```python
from build123d import *

# Parameters (mm, degrees)
BOSS_EXTRUDE1_DEPTH = 1.5


with BuildPart() as part:
    # Sketch2 → Boss-Extrude1 (new body, symmetric)
    with BuildSketch(Plane.XY):
        with BuildLine():
            Line((-15.000000098, -155.000001017), (-1.550000098, -155.000001017))
            Line((-1.550000098, -155.000001017), (-1.550000098, 164.999998983))
            Line((-1.550000098, 164.999998983), (1.549999902, 164.999998983))
            Line((1.549999902, 164.999998983), (1.549999902, -155.000001017))
            Line((1.549999902, -155.000001017), (14.999999902, -155.000001017))
            Line((14.999999902, -155.000001017), (14.999999902, 154.999998983))
            ThreePointArc((14.999999902, 154.999998983), (1.936e-06, 170.000001017), (-15.000000098, 155.000003052))
            Line((-15.000000098, 155.000003052), (-15.000000098, -155.000001017))
        make_face()
    extrude(amount=BOSS_EXTRUDE1_DEPTH, both=True)


solid = part.part
```
Part model, mm, in its own coordinate system. Give positions to 0.01 mm unless a question says otherwise; leave off trailing zeros. Write each loop counter-clockwise with the first axis right and the second up, starting at its lowest first coordinate (ties: lowest second). Pieces come first, ordered by that corner, then holes. Notation, with made-up numbers: (-10, 49.25) -> (7, 49.25) arc R14 cw to (7, 54.25) -> close; hole circle Ø10 at (53, 12.5). An arc over 180 degrees is marked (long way). Put each result on its own line as item: value. Start each with the question number.
Item 1: Cut at A-A (y = -106). List the corners of the cut face in (x, z), then the cut area to 3 significant figures.
Item 2: Cut at B-B (z = -1). List the corners of the cut face in (x, y), then the cut area to 3 significant figures.
Item 3: Pin check, flat tips, straight feed: pin 1 Ø1 at (x, z) = (-11.5, 0) entering from +Y; pin 2 Ø0.9 at (x, z) = (0.5, 0.5) entering from -Y. Stop position of each tip, or through.
Item 4: Wall check: L1, parallel to X at y = -88, z = 0.15; L2, parallel to Y at x = 0.5, z = 0.8; L3, parallel to Y at x = 3, z = 0.1. Give the ranges that are in metal, low to high. Write a range as [from, to].
Answer list:
1. outline: (-15, -1.5) -> (-1.55, -1.5) -> (-1.55, 1.5) -> (-15, 1.5) -> close; (1.55, -1.5) -> (15, -1.5) -> (15, 1.5) -> (1.55, 1.5) -> close
1. area: 80.7 mm2
2. outline: (-15, -155) -> (-1.55, -155) -> (-1.55, 165) -> (1.55, 165) -> (1.55, -155) -> (15, -155) -> (15, 155) arc R15 ccw to (-15, 155) -> close
2. area: 8,660 mm2
3. pin 1: stops at y = 165.2
3. pin 2: stops at y = 165
4. L1: x = [-15, -1.55], [1.55, 15]
4. L2: y = [165, 169.99]
4. L3: y = [-155, 169.7]
